Source: CAD feature listing. Evaluate the final solid. Frame: model axes, mm. A direction names the side the tool comes from. Coordinates: 2 decimals unless noted, no trailing zeros. Write each loop counter-clockwise with the first axis right and the second up, starting at its lowest first coordinate (ties: lowest second). Pieces come first, ordered by that corner, then holes. Notation, with made-up numbers: (88, 78) - (120, 78) arc R32 ccw to (120, 106) - close; hole circle Ø6 at (-39.5, 4). An arc over 180 degrees is marked (long way). One line per question, with ' | ' between items.
from build123d import *

# Parameters (mm, degrees)
F0_W     = 89
F0_H     = 55.5
F1_DEPTH = 3
F0_W_2   = 95
F0_H_2   = 61.5
F2_DEPTH = 16
F4_DEPTH = 95
F5_W     = 61.5
F5_H     = 3.5
F6_DEPTH = 3
F7_R     = 5
F8_R     = 2
F9_R     = 3


with BuildPart() as f1:
    # F0 (on Top) → F1 (new body)
    with BuildSketch(Plane.XY):
        Rectangle(F0_W, F0_H)
    extrude(amount=F1_DEPTH)

    # F0 (on Top) → F2 (join)
    with BuildSketch(Plane.XY):
        Rectangle(F0_W_2, F0_H_2)
        Rectangle(F0_W, F0_H, mode=Mode.SUBTRACT)
    extrude(amount=F2_DEPTH)

    # F3 (on face) → F4 (join, through all)
    with BuildSketch(Plane.YZ.offset(47.5)):
        Polygon((29.25, 16), (30.75, 16), (30.75, 19.5), (27.75, 19.5), (27.75, 17.2), (29.25, 17.2), align=None)
        Polygon((-29.25, 17.2), (-27.75, 17.2), (-27.75, 19.5), (-30.75, 19.5), (-30.75, 16), (-29.25, 16), align=None)
    extrude(amount=-F4_DEPTH)

    # F5 (on face) → F6 (join)
    with BuildSketch(Plane(origin=(-47.5, 0, 0), x_dir=(0, -1, 0), z_dir=(-1, 0, 0))):
        with Locations((0, 17.75)):
            Rectangle(F5_W, F5_H)
    extrude(amount=-F6_DEPTH)

    # F7
    f7_edges = [f1.edges().sort_by_distance(p)[0] for p in [
        (47.5, -30.75, 9.75),
        (-47.5, -30.75, 9.75),
        (47.5, 30.75, 9.75),
        (-47.5, 30.75, 9.75),
    ]]
    fillet(f7_edges, radius=F7_R)

    # F8
    f8_edges = [f1.edges().sort_by_distance(p)[0] for p in [
        (-44.5, 27.75, 9.5),
        (-44.5, -27.75, 9.5),
        (44.5, -27.75, 9.5),
        (44.5, 27.75, 9.5),
    ]]
    fillet(f8_edges, radius=F8_R)

    # F9
    f9_edges = [f1.edges().sort_by_distance(p)[0] for p in [
        (-44.5, -29.25, 16.6),
        (-44.5, 29.25, 16.6),
    ]]
    fillet(f9_edges, radius=F9_R)


solid = f1.part
Item 1: Mould query, pull axis Y, two halves, no side actions, for faces 5 (the face through (-1, -30.75, 10)), 6 (the face through (-1, -27.75, 9)), 7 (the face through (-47.5, 0, 10)). Classes: pulls with the +Y half, pulls with the -Y half, needs draft (parallel to the pull), parting line crosses it, or undercut.
Check sheet entries:
face 5: pulls with the -Y half | face 6: undercut | face 7: needs draft
Item 2: Cut plane C-C on y = -18. Return loops of the section in (x, z).
Check sheet entries:
outline: (-47.5, 0) - (47.5, 0) - (47.5, 16) - (44.5, 16) - (44.5, 3) - (-44.5, 3) - (-44.5, 19.5) - (-47.5, 19.5) - close
Item 3: Access query for faces 1 (the face through (15, -28, 16)), 2 (the face through (-1, 0, 0)), 3 (the face through (2, 27.75, 18)), 4 (the face through (-43.93, -27.15, 9.59)). Directions: +Z, -Z, +X, -X, +Y, -Y. A direction counts if a zero-diameter tool reaches every point of the face in a straight line with its end or side. Return the directions, or none.
Check sheet entries:
face 1: +X | face 2: -Z, +X, -X, +Y, -Y | face 3: +Z, +X | face 4: +Z
Item 4: Ray query, line 1 along X through (y, z) = (-17, 3.75); line 2 along Y through (x, z) = (-29, 17.25); line 3 along Z through (x, y) = (-21, 13). Return the intervals inside material, ascending. Write a range as [from, to].
Check sheet entries:
line 1: [-47.5, -44.5], [44.5, 47.5] | line 2: [-30.75, -27.75], [27.75, 30.75] | line 3: [0, 3]
Item 5: Pin query (flat end, axial travel): pin 1 Ø17.5 at (x, y) = (-14, 3.5) entering from +Z; pin 2 Ø0.8 at (x, y) = (-19, -28.5) entering from -Z. Return the tip coordinate at first contact, or that it passes through.
Check sheet entries:
pin 1: z = 3 | pin 2: z = 0
Item 6: Cut plane B-B on x = 11. Return loops of the section in (y, z), and give its area (3 significant figures).
Check sheet entries:
outline: (-30.75, 0) - (30.75, 0) - (30.75, 19.5) - (27.75, 19.5) - (27.75, 17.2) - (29.25, 17.2) - (29.25, 16) - (27.75, 16) - (27.75, 3) - (-27.75, 3) - (-27.75, 16) - (-29.25, 16) - (-29.25, 17.2) - (-27.75, 17.2) - (-27.75, 19.5) - (-30.75, 19.5) - close | area: 280 mm²
Item 7: Cut plane A-A on z = 5.5. Return loops of the section in (x, y), and give its area (3 significant figures).
Check sheet entries:
outline: (-47.5, -25.75) arc R5 ccw to (-42.5, -30.75) - (42.5, -30.75) arc R5 ccw to (47.5, -25.75) - (47.5, 25.75) arc R5 ccw to (42.5, 30.75) - (-42.5, 30.75) arc R5 ccw to (-47.5, 25.75) - close; hole (-44.5, -25.75) arc R2 ccw to (-42.5, -27.75) - (42.5, -27.75) arc R2 ccw to (44.5, -25.75) - (44.5, 25.75) arc R2 ccw to (42.5, 27.75) - (-42.5, 27.75) arc R2 ccw to (-44.5, 25.75) - close | area: 885 mm²
